For this review, take the finished solid that the model builds, in its own axes (mm). A direction names the side the tool comes from. Round coordinates to 2 decimals unless told otherwise and drop trailing zeros. Write each loop counter-clockwise with the first axis right and the second up, starting at its lowest first coordinate (ties: lowest second). Pieces come first, ordered by that corner, then holes. Notation, with made-up numbers: (26, 37.5) - (56, 37.5) arc R18 cw to (56, 70.5) - close; hole circle Ø8 at (-13.5, 75.5). An arc over 180 degrees is marked (long way). One line per item, written item: value. Start each with the question number.
Q1. Clearance check with flat-ended pins moving along their axes: pin 1 Ø10 at (x, z) = (11, 7.5) entering from -Y; pin 2 Ø10 at (x, y) = (48, -6) entering from +Z; pin 3 Ø12 at (x, z) = (22.5, -7.5) entering from +Y. State where each tip first meets the part, or that it passes through.
Q2. Add section C-C on x = 7. Write out the cut boundary in (y, z), and give its area (3 significant figures).
Q3. Tool access review of faces 1 (the face through (30.506, 11.923, 3.755)), 2 (the face through (37.805, -0.1, 10.2)), 3 (the face through (23, -0.1, 10.2)): name each direction out of +Z, -Z, +X, -X, +Y, -Y from which nothing blocks a thin tool from reaching the whole face with its end or side.
Q4. Add section B-B on z = 1.25. Write out the cut boundary in (x, y) (3 decimals), and give its area (3 significant figures).
Q5. Add section A-A on y = 0. Write out the cut boundary in (x, z) (3 decimals), and give its area (3 significant figures).
Q6. For probe 1 along X at (y, z) = (11.25, 4.5) (3 decimals); probe 2 along Y at (x, z) = (14.5, -0.5); probe 3 along Z at (x, y) = (24.5, 0), list the stretches that pass through material, from the lowest coordinate up.
Autodesk Inventor part; units mm, degrees
ref_plane "YZ Plane" through (0, 0, 0) normal (1, 0, 0) x (0, 1, 0)
ref_plane "XZ Plane" through (0, 0, 0) normal (0, 1, 0) x (-1, 0, 0)
ref_plane "XY Plane" through (0, 0, 0) normal (0, 0, 1) x (1, 0, 0)
sketch "Эскиз1" plane through (0, 0, 0) normal (0, 0, 1) x (1, 0, 0)
  line L0 (0, 0) -> (53.555, 0)
  line L1 (0, 0) -> (0, 10)
  line L2 (37.805, 12.5) -> (37.805, 10)
  line L3 (37.805, 10) -> (53.555, 10)
  line L4 (53.555, 10) -> (53.555, 0)
  line L5 (2, 10) -> (2, 10)
  line L6 (2, 10) -> (23, 10)
  line L7 (23, 10) -> (23, 12.5)
  line L8 (0, 10) -> (2, 10)
  line L9 (23, 12.5) -> (37.805, 12.5)
  dimension "d0" = 20
  dimension "d2" = 15.75
  dimension "d5" = 20
  dimension "d6" = 21
  dimension "d7" = 2
  dimension "d8" = 20
  dimension "d9" = 25
  dimension "d10" = 37.805
revolve "Вращение1" add sketch "Эскиз1" angle 360 about axis through (0, 0, 0) along (1, 0, 0)
properties part number "Валл_резина"
Result set:
1. pin 1: stops at y = -9.68
1. pin 2: stops at z = 9.95
1. pin 3: stops at y = 12.41
2. outline: circle Ø20 at (0, 0)
2. area: 314 mm^2
3. face 1: +X, -X
3. face 2: +X
3. face 3: -X
4. outline: (0, -9.922) - (23, -9.922) - (23, -12.437) - (37.805, -12.437) - (37.805, -9.922) - (53.555, -9.922) - (53.555, 9.922) - (37.805, 9.922) - (37.805, 12.437) - (23, 12.437) - (23, 9.922) - (0, 9.922) - close
4. area: 1,140 mm^2
5. outline: (0, -10) - (23, -10) - (23, -12.5) - (37.805, -12.5) - (37.805, -10) - (53.555, -10) - (53.555, 10) - (37.805, 10) - (37.805, 12.5) - (23, 12.5) - (23, 10) - (0, 10) - close
5. area: 1,150 mm^2
6. probe 1: x = 23 to 37.805
6. probe 2: y = -9.99 to 9.99
6. probe 3: z = -12.5 to 12.5
